For this review, take the finished solid that the model builds, in its own axes (mm). A direction names the side the tool comes from. Round coordinates to 2 decimals unless told otherwise and drop trailing zeros. Write each loop counter-clockwise with the first axis right and the second up, starting at its lowest first coordinate (ties: lowest second). Pieces come first, ordered by that corner, then holes.
from build123d import *

# Parameters (mm, degrees)
SKETCH1_R           = 12.5
BOSS_EXTRUDE1_DEPTH = 110
SKETCH2_R           = 22.5
BOSS_EXTRUDE2_DEPTH = 10
BOSS_EXTRUDE2_TAPER = 30
SKETCH3_R           = 4
CUT_EXTRUDE1_DEPTH  = 30


with BuildPart() as part:
    # Sketch1 → Boss-Extrude1 (new body)
    with BuildSketch(Plane(origin=(0, 0, 0), x_dir=(1, 0, 0), z_dir=(0, 1, 0))):
        with Locations(Location((0, 0, 0), (0, 0, 270))):
            Circle(SKETCH1_R)
    extrude(amount=BOSS_EXTRUDE1_DEPTH)

    # Sketch2 → Boss-Extrude2 (add)
    with BuildSketch(Plane(origin=(0, 110, 0), x_dir=(1, 0, 0), z_dir=(0, 1, 0))):
        Circle(SKETCH2_R)
    extrude(amount=BOSS_EXTRUDE2_DEPTH, taper=BOSS_EXTRUDE2_TAPER)

    # Sketch3 → Cut-Extrude1 (cut, symmetric)
    with BuildSketch(Plane.XY):
        with Locations(Location((0, 12, 0), (0, 0, 89.99999999))):
            Circle(SKETCH3_R)
    extrude(amount=CUT_EXTRUDE1_DEPTH, both=True, mode=Mode.SUBTRACT)


solid = part.part
(1) For line 1 along Z through (x, y) = (-0.5, 87.5); line 2 along X through (y, z) = (35, 0); line 3 along X through (y, z) = (12, -2.5), list the stretches that pass through material, from the lowest coordinate up.
Geometry check:
line 1: z = -12.49 to 12.49
line 2: x = -12.5 to 12.5
line 3: x = -12.25 to -4, 4 to 12.25
(2) For faces 1 (the face through (0, 0, 0)), 2 (the face through (3.755, 54.23, 11.923)), list the 3-axis set-ups (+Z, -Z, +X, -X, +Y, -Y) from which the entire face can be reached by the end or side of a thin tool; tool diameter is ignored.
Geometry check:
face 1: +Z, -Z, +X, -X, -Y
face 2: -Y
(3) We need section B-B, the plane y = 11. Give the boundary of the cut face in (x, z), and give its area (3 significant figures).
Geometry check:
outline: (-3.87, -11.88) - (-3.87, 11.88) arc R12.5 ccw to start; (3.87, -11.88) arc R12.5 ccw to (3.87, 11.88) - close
area: 300 mm2
(4) Mouldability with a two-part tool opening along X and no side actions: class faces 3 (the face through (16.221, 119.514, -5.108)), 4 (the face through (0, 120, 0)), 5 (the face through (0, 8, 0)) as pulls with the +X half, pulls with the -X half, needs draft (parallel to the pull), parting line crosses it, or undercut.
Geometry check:
face 3: parting line crosses it
face 4: needs draft
face 5: undercut
(5) We need section A-A, the plane x = 0. Give the boundary of the cut face in (y, z).
Geometry check:
outline: (0, -12.5) - (8, -12.5) - (8, 12.5) - (0, 12.5) - close; (16, -12.5) - (110, -12.5) - (110, -22.5) - (120, -16.73) - (120, 16.73) - (110, 22.5) - (110, 12.5) - (16, 12.5) - close
(6) We need section C-C, the plane y = 29. Give the boundary of the cut face in (x, z), and give its area (3 significant figures).
Geometry check:
outline: circle Ø25 at (0, 0)
area: 491 mm2
(7) For pin 1 Ø6 at (y, z) = (37.5, -4.5) entering from -X; pin 2 Ø6 at (y, z) = (42, 4) entering from -X; pin 3 Ø10.5 at (x, y) = (0, 12) entering from -Z, all flat-tipped, find the tip position at first contact; note any pin that passes through.
Geometry check:
pin 1: stops at x = -12.41
pin 2: stops at x = -12.46
pin 3: stops at z = -12.5
